The model under review builds one solid part; all positions refer to its coordinate system, in mm. Face numbers are marked on the shaded views. A direction names the side the tool comes from. Coordinates: 2 decimals unless noted, no trailing zeros. Loops run counter-clockwise (first coordinate to the right, second up) from the corner with the lowest first, then second, coordinate; pieces in that order, holes last. Notation, with made-up numbers: M -1.5,52 L 34.5,52 A21 ccw 34.5,69 Z; hole C -1.75,15 d9. An arc over 180 degrees is marked long. Return JSON: item names as keys, results as strings.
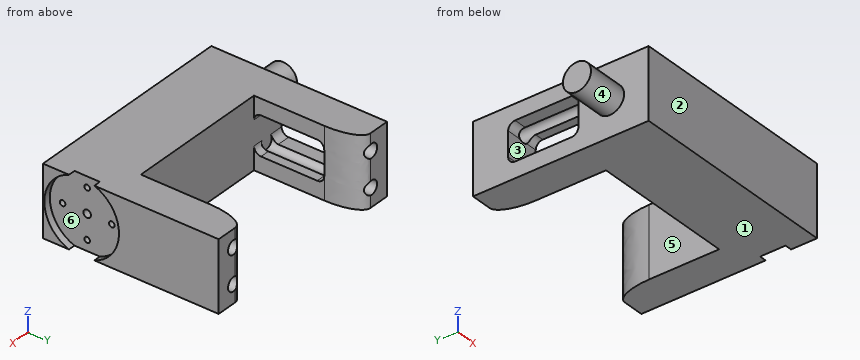
```python
from build123d import *

# Parameters (mm, degrees)
SKIZZE1_W                       = 61
SKIZZE1_H                       = 50
AUFSATZ_LINEAR_AUSTRAGEN1_DEPTH = 20
SKIZZE2_W                       = 41
SKIZZE2_H                       = 20
SCHNITT_LINEAR_AUSTRAGEN1_DEPTH = 30
SCHNITT_LINEAR_START            = -61
SKIZZE3_W                       = 11
SKIZZE3_H                       = 20
SCHNITT_LINEAR_AUSTRAGEN2_DEPTH = 10
SCHNITT_LINEAR_AUSTRAGEN3_REACH = 83.37
SKIZZE4_R                       = 1.95
VERRUNDUNG1_SIZE                = 4
VERRUNDUNG1_SIZE_2              = 10
VERRUNDUNG2_R                   = 2
SKIZZE6_R                       = 10.631095309
SCHNITT_LINEAR_AUSTRAGEN4_DEPTH = 2
SKIZZE7_R                       = 0.8
SCHNITT_LINEAR_AUSTRAGEN5_DEPTH = 22
SKIZZE10_R                      = 1.095488433
SCHNITT_LINEAR_AUSTRAGEN6_DEPTH = 63
SKIZZE11_R                      = 4
AUFSATZ_LINEAR_AUSTRAGEN3_DEPTH = 12


with BuildPart() as part:
    # Skizze1 → Aufsatz-Linear austragen1 (new body)
    with BuildSketch(Plane.XY):
        with Locations((30.5, 25)):
            Rectangle(SKIZZE1_W, SKIZZE1_H)
    extrude(amount=AUFSATZ_LINEAR_AUSTRAGEN1_DEPTH)

    # Skizze2 → Schnitt-Linear austragen1 (cut)
    with BuildSketch(Plane(origin=(0, 50, 0), x_dir=(1, 0, 0), z_dir=(0, 1, 0))):
        with Locations((30.5, -10)):
            Rectangle(SKIZZE2_W, SKIZZE2_H)
    extrude(amount=-SCHNITT_LINEAR_AUSTRAGEN1_DEPTH, mode=Mode.SUBTRACT)

    # Skizze3 → Schnitt-Linear austragen2 (cut)
    with BuildSketch(Plane(origin=(61, 0, 0), x_dir=(0, 0, -1), z_dir=(1, 0, 0)).offset(SCHNITT_LINEAR_START)):
        with Locations((-10, 30)):
            Rectangle(SKIZZE3_W, SKIZZE3_H)
    extrude(amount=SCHNITT_LINEAR_AUSTRAGEN2_DEPTH, mode=Mode.SUBTRACT)

    # Schnitt-Linear austragen3: up to this face of the body (flat: up to its plane)
    schnitt_linear_austragen3_end = Plane(part.part.faces().sort_by_distance((27.483870968, 20, 10))[0])
    # Skizze4 → Schnitt-Linear austragen3 (cut, up to the picked face)
    with BuildSketch(Plane(origin=(0, 50, 0), x_dir=(1, 0, 0), z_dir=(0, 1, 0)), mode=Mode.PRIVATE) as schnitt_linear_austragen3_sk1:
        with Locations(Location((5.54, -5.225, 0), (0, 0, 270))):
            Circle(SKIZZE4_R)
    schnitt_linear_austragen3_tool1 = split(extrude(schnitt_linear_austragen3_sk1.sketch, amount=-SCHNITT_LINEAR_AUSTRAGEN3_REACH, mode=Mode.PRIVATE), bisect_by=schnitt_linear_austragen3_end, keep=Keep.BOTH, mode=Mode.PRIVATE)
    # Skizze4 → Schnitt-Linear austragen3 (cut, up to the picked face)
    with BuildSketch(Plane(origin=(0, 50, 0), x_dir=(1, 0, 0), z_dir=(0, 1, 0)), mode=Mode.PRIVATE) as schnitt_linear_austragen3_sk2:
        with Locations(Location((5.54, -15.075, 0), (0, 0, 270))):
            Circle(SKIZZE4_R)
    schnitt_linear_austragen3_tool2 = split(extrude(schnitt_linear_austragen3_sk2.sketch, amount=-SCHNITT_LINEAR_AUSTRAGEN3_REACH, mode=Mode.PRIVATE), bisect_by=schnitt_linear_austragen3_end, keep=Keep.BOTH, mode=Mode.PRIVATE)
    # Skizze4 → Schnitt-Linear austragen3 (cut, up to the picked face)
    with BuildSketch(Plane(origin=(0, 50, 0), x_dir=(1, 0, 0), z_dir=(0, 1, 0)), mode=Mode.PRIVATE) as schnitt_linear_austragen3_sk3:
        with Locations(Location((55.66, -15.075, 0), (0, 0, 270))):
            Circle(SKIZZE4_R)
    schnitt_linear_austragen3_tool3 = split(extrude(schnitt_linear_austragen3_sk3.sketch, amount=-SCHNITT_LINEAR_AUSTRAGEN3_REACH, mode=Mode.PRIVATE), bisect_by=schnitt_linear_austragen3_end, keep=Keep.BOTH, mode=Mode.PRIVATE)
    # Skizze4 → Schnitt-Linear austragen3 (cut, up to the picked face)
    with BuildSketch(Plane(origin=(0, 50, 0), x_dir=(1, 0, 0), z_dir=(0, 1, 0)), mode=Mode.PRIVATE) as schnitt_linear_austragen3_sk4:
        with Locations(Location((55.66, -5.225, 0), (0, 0, 270))):
            Circle(SKIZZE4_R)
    schnitt_linear_austragen3_tool4 = split(extrude(schnitt_linear_austragen3_sk4.sketch, amount=-SCHNITT_LINEAR_AUSTRAGEN3_REACH, mode=Mode.PRIVATE), bisect_by=schnitt_linear_austragen3_end, keep=Keep.BOTH, mode=Mode.PRIVATE)
    add(schnitt_linear_austragen3_tool1.solids().sort_by(Axis((5.54, 50, 5.225), (0, -1, 0)))[0], mode=Mode.SUBTRACT)
    add(schnitt_linear_austragen3_tool2.solids().sort_by(Axis((5.54, 50, 15.075), (0, -1, 0)))[0], mode=Mode.SUBTRACT)
    add(schnitt_linear_austragen3_tool3.solids().sort_by(Axis((55.66, 50, 15.075), (0, -1, 0)))[0], mode=Mode.SUBTRACT)
    add(schnitt_linear_austragen3_tool4.solids().sort_by(Axis((55.66, 50, 5.225), (0, -1, 0)))[0], mode=Mode.SUBTRACT)

    # Verrundung1
    # an asymmetric fillet: 10, 4 mm, written as the material it takes off along each edge
    with BuildSketch(Plane(origin=(51, 50, -25), x_dir=(1, 0, 0), z_dir=(0, 0, 1)), Plane(origin=(10, 50, 45), x_dir=(-1, 0, 0), z_dir=(0, 0, -1))) as verrundung1_piece_1:
        with BuildLine():
            Bezier((VERRUNDUNG1_SIZE, 0), (0, 0), (0, -VERRUNDUNG1_SIZE_2), weights=[1, 0.707106781, 1])
            Line((0, -VERRUNDUNG1_SIZE_2), (0, 0))
            Line((0, 0), (VERRUNDUNG1_SIZE, 0))
        make_face()
    extrude(amount=70, mode=Mode.SUBTRACT)

    # Verrundung2
    verrundung2_edges = [part.edges().sort_by_distance(p)[0] for p in [
        (1.818438783, 40, 15.5),
        (8.721561217, 40, 15.5),
        (8.675107038, 40, 4.5),
        (1.864892962, 40, 4.5),
        (8.721561217, 20, 15.5),
        (1.818438783, 20, 15.5),
        (8.675107038, 20, 4.5),
        (1.864892962, 20, 4.5),
    ]]
    fillet(verrundung2_edges, radius=VERRUNDUNG2_R)

    # Skizze6 → Schnitt-Linear austragen4 (cut)
    with BuildSketch(Plane(origin=(61, 0, 0), x_dir=(0, 0, -1), z_dir=(1, 0, 0))):
        with Locations((-10, 11)):
            Circle(SKIZZE6_R)
    extrude(amount=-SCHNITT_LINEAR_AUSTRAGEN4_DEPTH, mode=Mode.SUBTRACT)

    # Skizze7 → Schnitt-Linear austragen5 (cut)
    with BuildSketch(Plane(origin=(59, 0, 0), x_dir=(0, 0, -1), z_dir=(1, 0, 0))):
        with Locations(Location((-10, 18, 0), (0, 0, 90))):
            Circle(SKIZZE7_R)
        with Locations(Location((-3, 11, 0), (0, 0, 90))):
            Circle(SKIZZE7_R)
        with Locations(Location((-10, 4, 0), (0, 0, 90))):
            Circle(SKIZZE7_R)
        with Locations(Location((-17, 11, 0), (0, 0, 90))):
            Circle(SKIZZE7_R)
    extrude(amount=-SCHNITT_LINEAR_AUSTRAGEN5_DEPTH, mode=Mode.SUBTRACT)

    # Skizze10 → Schnitt-Linear austragen6 (cut)
    with BuildSketch(Plane(origin=(59, 0, 0), x_dir=(0, 0, -1), z_dir=(1, 0, 0))):
        with Locations(Location((-10, 11, 0), (0, 0, 90))):
            Circle(SKIZZE10_R)
    extrude(amount=-SCHNITT_LINEAR_AUSTRAGEN6_DEPTH, mode=Mode.SUBTRACT)

    # Skizze11 → Aufsatz-Linear austragen3 (add)
    with BuildSketch(Plane.ZY):
        with Locations(Location((10, 11, 0), (0, 0, 90))):
            Circle(SKIZZE11_R)
    extrude(amount=AUFSATZ_LINEAR_AUSTRAGEN3_DEPTH)


solid = part.part
```
1. To check wall thickness, follow line 1 (X direction, y = 34, z = 16.25); line 2 (X direction, y = 31, z = 5); line 3 (Z direction, x = 29.5, y = 11). State the ranges of each line that lie inside material, in increasing order.
Check values:
{"line 1": "0 to 3.98, 7.1 to 10, 51 to 54.1, 57.22 to 61", "line 2": "51 to 53.72, 57.6 to 61", "line 3": "0 to 8.9, 11.1 to 20"}
2. Machinability: for the marked faces 4, 5 and 6, which of the approach directions +Z, -Z, +X, -X, +Y, -Y give a long, thin tool a straight path to every point of the face, cutting with its end or side? Answer none if there is none.
Check values:
{"face 4": "-X", "face 5": "+Z, -Z, +Y", "face 6": "+X"}
3. Add section B-B on x = 47.5. Give the boundary of the cut face in (y, z), plus the area to 3 significant figures.
Check values:
{"outline": "M 0,0 L 20,0 L 20,20 L 0,20 Z; hole C 4,10 d1.6; hole C 11,10 d2.19; hole C 11,3 d1.6; hole C 11,17 d1.6; hole C 18,10 d1.6", "area": "388 mm²"}
4. Add section C-C on x = 21. Give the boundary of the cut face in (y, z), plus the area to 3 significant figures.
Check values:
{"outline": "M 0,0 L 20,0 L 20,20 L 0,20 Z; hole C 11,10 d2.19", "area": "396 mm²"}
5. Add section D-D on x = -4. Give the boundary of the cut face in (y, z).
Check values:
{"outline": "C 11,10 d8"}
6. Insertion check: pin 1 Ø3 at (y, z) = (27, 13) entering from -X; pin 2 Ø2 at (y, z) = (11, 17) entering from +X; pin 3 Ø1.5 at (x, z) = (17, 12.5) entering from +Y. Each pin has a flat end and moves straight along its axis. Give the tip position at first contact, or say it passes through.
Check values:
{"pin 1": "x = 51", "pin 2": "x = 59", "pin 3": "y = 20"}
7. Add section A-A on y = 27. Give the boundary of the cut face in (x, z) (3 decimals), plus the area to 3 significant figures.
Check values:
{"outline": "M 0,0 L 10,0 L 10,4.5 L 7.35,4.5 A1.95 cw 3.73,4.5 L 0,4.5 Z; M 0,15.5 L 3.637,15.5 A1.95 cw 7.443,15.5 L 10,15.5 L 10,20 L 0,20 Z; M 51,0 L 61,0 L 61,20 L 51,20 Z; hole C 55.66,5.225 d3.9; hole C 55.66,15.075 d3.9", "area": "259 mm²"}
8. The part is to be moulded in two halves that separate along Z. For the marked faces 1, 2 and 3, say which applies: released by +Z, released by -Z, zero draft, split by the parting line, or undercut.
Check values:
{"face 1": "released by -Z", "face 2": "zero draft", "face 3": "undercut"}
